Input: part model. Units: mm. Frame: model coordinates. A direction names the side the tool comes from. Round coordinates to 2 decimals unless told otherwise and drop trailing zeros. Order: outer loops, then holes, each group sorted by start corner. A loop starts at its lowest first (then second) coordinate and runs counter-clockwise, first axis right, second up. Notation, with made-up numbers: (82.25, 51) -> (90.25, 51) arc R18 cw to (90.25, 59) -> close; hole circle Ø4 at (3.5, 6.25). An arc over 180 degrees is marked (long way). Use a Markdown table: item, result.
from build123d import *

# Parameters (mm, degrees)
BOSS_EXTRUDE1_DEPTH = 63.5
SKETCH2_R           = 2.9972
CUT_EXTRUDE1_DEPTH  = 12.7
SKETCH3_R           = 3.96875
CUT_EXTRUDE2_DEPTH  = 12.7
SKETCH4_R           = 1.27
CUT_EXTRUDE3_DEPTH  = 5.08


with BuildPart() as part:
    # Sketch1 → Boss-Extrude1 (new body)
    with BuildSketch(Plane.XY):
        Polygon((5.08, 0), (2.54, 4.399409051), (-2.54, 4.399409051), (-5.08, 0), (-2.54, -4.399409051), (2.54, -4.399409051), align=None)
    extrude(amount=BOSS_EXTRUDE1_DEPTH)

    # Sketch2 → Cut-Extrude1 (cut)
    with BuildSketch(Plane.XY.offset(63.5)):
        Circle(SKETCH2_R)
    extrude(amount=-CUT_EXTRUDE1_DEPTH, mode=Mode.SUBTRACT)

    # Sketch3 → Cut-Extrude2 (cut)
    with BuildSketch(Plane(origin=(0, 0, 0), x_dir=(-1, 0, 0), z_dir=(0, 0, -1))):
        Polygon((5.08, 0), (2.54, 4.399409051), (-2.54, 4.399409051), (-5.08, 0), (-2.54, -4.399409051), (2.54, -4.399409051), align=None)
        Circle(SKETCH3_R, mode=Mode.SUBTRACT)
    extrude(amount=-CUT_EXTRUDE2_DEPTH, mode=Mode.SUBTRACT)

    # Sketch4 → Cut-Extrude3 (cut)
    with BuildSketch(Plane(origin=(-3.81, 2.199704526, 0), x_dir=(0, 0, 1), z_dir=(-0.8660254037844385, 0.5000000000000004, 0))):
        with Locations(Location((57.15, 0, 0), (0, 0, 270))):
            Circle(SKETCH4_R)
    extrude(amount=-CUT_EXTRUDE3_DEPTH, mode=Mode.SUBTRACT)


solid = part.part
1) Pull-direction query (Y, two-part tool) for faces 4 (the cylindrical face through (-3.696, 0.735, 57.531)), 5 (the flat face through (0, 4.399, 38)), 6 (the flat face through (0, -4.399, 38)); classes: +Y half, -Y half, draft (parallel to the pull), parting line (faces both ways), or undercut.
Results found:
| item | result |
|---|---|
| face 4 | undercut |
| face 5 | +Y half |
| face 6 | -Y half |
2) Cut plane A-A on x = 0. Return loops of the section in (y, z), and give its area (3 significant figures).
Results found:
| item | result |
|---|---|
| outline | (-4.4, 12.7) -> (-3.97, 12.7) -> (-3.97, 0) -> (3.97, 0) -> (3.97, 12.7) -> (4.4, 12.7) -> (4.4, 63.5) -> (3, 63.5) -> (3, 50.8) -> (-3, 50.8) -> (-3, 63.5) -> (-4.4, 63.5) -> close |
| area | 472 mm² |
3) Set-up query: faces 1 (the flat face through (0, 0, 0)), 2 (the cylindrical face through (0.86, -3.874, 6.261)), 3 (the cylindrical face through (2.769, -1.148, 57.239)). Return all of +Z, -Z, +X, -X, +Y, -Y with unobstructed straight access to the full face (end or side cutting, diameter ignored); none if empty.
Results found:
| item | result |
|---|---|
| face 1 | -Z, +X, -X, +Y, -Y |
| face 2 | -Z |
| face 3 | +Z |
4) Cut plane C-C on z = 5. Return loops of the section in (x, y).
Results found:
| item | result |
|---|---|
| outline | circle Ø7.94 at (0, 0) |
5) Cut plane B-B on z = 30. Return loops of the section in (x, y), and give its area (3 significant figures).
Results found:
| item | result |
|---|---|
| outline | (-5.08, 0) -> (-2.54, -4.4) -> (2.54, -4.4) -> (5.08, 0) -> (2.54, 4.4) -> (-2.54, 4.4) -> close |
| area | 67.0 mm² |
6) Line query: L1, parallel to Y at x = 0, z = 59.5; L2, parallel to Z at x = 3.75, y = -2; L3, parallel to Z at x = -3.25, y = 3. Output: solid intervals per line, ascending. Write a range as [from, to].
Results found:
| item | result |
|---|---|
| L1 | y = [-4.4, -3], [3, 4.4] |
| L2 | z = [12.7, 63.5] |
| L3 | z = [12.7, 56.33], [57.97, 63.5] |
